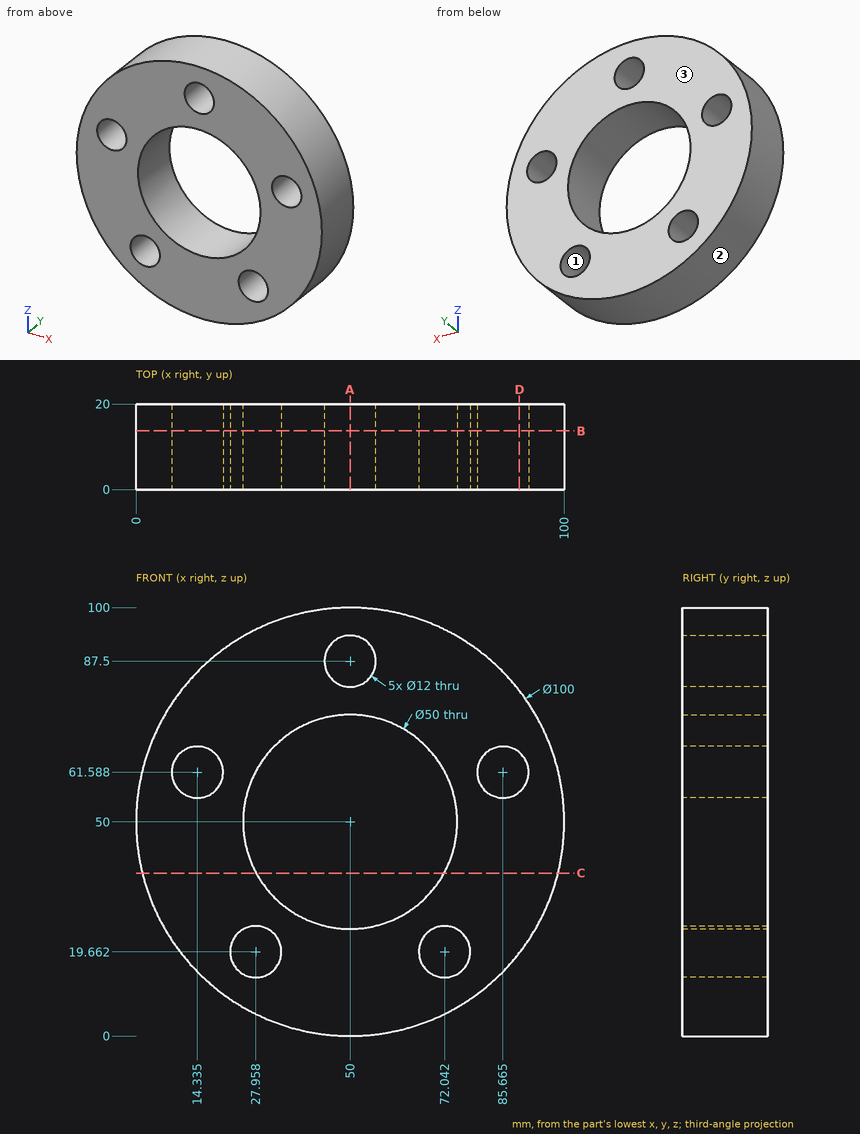
Design review of the part shown in the three views and the two pictorial views. Dimensions are in mm from the part's minimum x, y and z. Coordinates: 2 decimals unless noted, no trailing zeros. Order: outer loops, then holes, each group sorted by start corner. A loop starts at its lowest first (then second) coordinate and runs counter-clockwise, first axis right, second up. Notation, with made-up numbers: (-2, -23) -> (19, -23) arc R18 cw to (19, 11) -> close; hole circle Ø3 at (72.5, -29). An arc over 180 degrees is marked (long way). Use one line per item in the form item = value. Start each with the question number.
(1) Add section A-A on x = 50. State the section outline as (y, z) points, plus the area to 3 significant figures.
(2) Add section D-D on x = 89.5. State the section outline as (y, z) points (1 decimal), plus the area to 3 significant figures.
(3) For probe 1 along Z at (x, y) = (50, 7); probe 2 along X at (y, z) = (4.5, 21.5) (1 decimal); probe 3 along X at (y, z) = (14, 60.5) (1 decimal), list the stretches that pass through material, from the lowest coordinate up.
(4) Insertion check: pin 1 (10 mm diameter, centred on y = 7.5, z = 40.5, fed in from -X); pin 2 (12 mm diameter, centred on x = 73, y = 14.5, fed in from -Z); pin 3 (1 mm diameter, centred on y = 2.5, z = 63, fed in from +X); pin 4 (6 mm diameter, centred on x = 32.5, z = 72, fed in from -Y). Each pin has a flat end and moves straight along its axis. Give the tip position at first contact, or say it passes through.
(5) Add section B-B on y = 13.75. State the section outline as (x, z) points (1 decimal).
(6) Add section C-C on z = 38. State the section outline as (x, y) points, plus the area to 3 significant figures.
(7) The part is to be moulded in two halves that separate along X. For the marked faces 1, 2 and 3, say which applies: +X half, -X half, draft (parallel to the pull), parting line (faces both ways), or undercut.
Answer block:
q1.outline = (0, 0) -> (20, 0) -> (20, 25) -> (0, 25) -> close; (0, 75) -> (20, 75) -> (20, 81.5) -> (0, 81.5) -> close; (0, 93.5) -> (20, 93.5) -> (20, 100) -> (0, 100) -> close
q1.area = 760 mm²
q2.outline = (0, 19.3) -> (20, 19.3) -> (20, 57) -> (0, 57) -> close; (0, 66.2) -> (20, 66.2) -> (20, 80.7) -> (0, 80.7) -> close
q2.area = 1,040 mm²
q3.probe_1 = 0 to 25, 75 to 81.5, 93.5 to 100
q3.probe_2 = 8.9 to 22.2, 33.7 to 66.3, 77.8 to 91.1
q3.probe_3 = 1.1 to 8.4, 20.2 to 27.3, 72.7 to 79.8, 91.6 to 98.9
q4.pin_1 = 0.2
q4.pin_2 = 2.98
q4.pin_3 = 98.41
q4.pin_4 = 0
q5.outline = circle Ø100 at (50, 50); hole circle Ø12 at (14.3, 61.6); hole circle Ø12 at (28, 19.7); hole circle Ø50 at (50, 50); hole circle Ø12 at (50, 87.5); hole circle Ø12 at (72, 19.7); hole circle Ø12 at (85.7, 61.6)
q6.outline = (1.46, 0) -> (28.07, 0) -> (28.07, 20) -> (1.46, 20) -> close; (71.93, 0) -> (98.54, 0) -> (98.54, 20) -> (71.93, 20) -> close
q6.area = 1,060 mm²
q7.face_1 = undercut
q7.face_2 = parting line
q7.face_3 = draft
